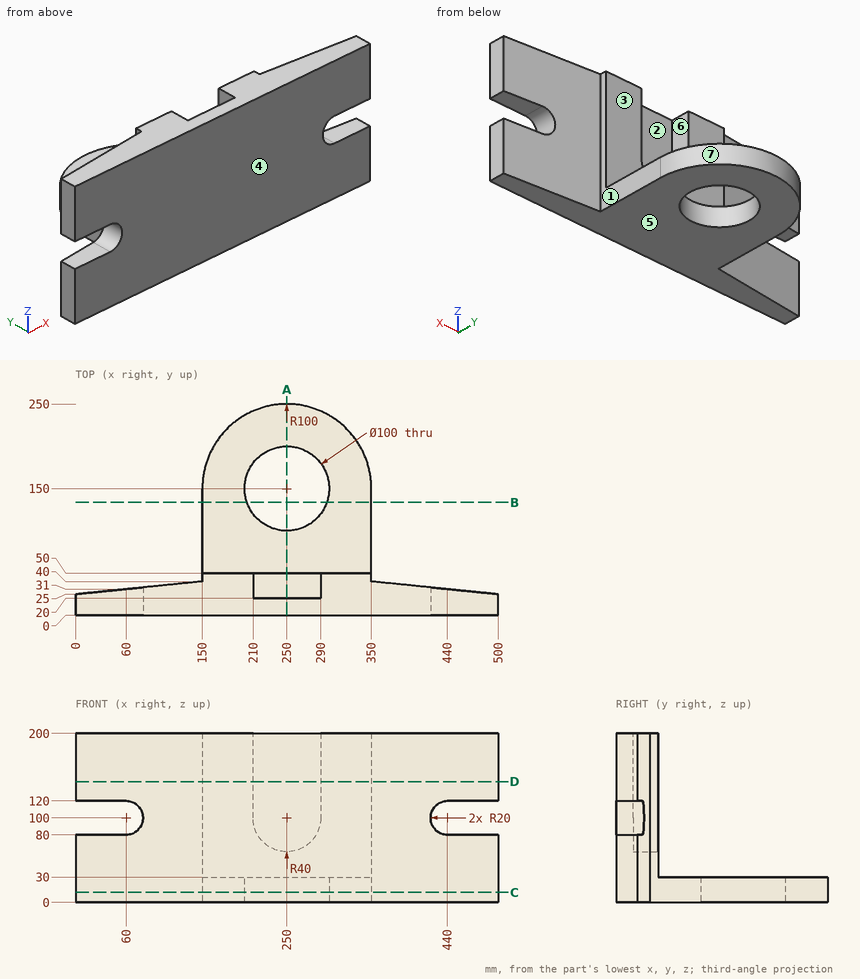
Here's the drawing with two shaded views (mm, measured from the low corner). I have some questions. A direction names the side the tool comes from. Give positions to 0.01 mm unless a question says otherwise; leave off trailing zeros. Write each loop counter-clockwise with the first axis right and the second up, starting at its lowest first coordinate (ties: lowest second). Pieces come first, ordered by that corner, then holes. Notation, with made-up numbers: (-23, 33) - (1, 33) arc R27 ccw to (1, 49) - close; hole circle Ø1 at (42, 55). An arc over 180 degrees is marked (long way). One line per item, written item: value. Start each with the question number.
Item 1: I'm going to push flat-ended pins straight in: pin 1 (8 mm diameter, centred on y = 68.5, z = 29.5, fed in from +X); pin 2 (3 mm diameter, centred on x = 187.5, z = 29.5, fed in from +Y). Where does each tip first touch, or does it pass through?
Item 2: Which directions (+Z, -Z, +X, -X, +Y, -Y) give clear straight access to the entire face, cutting with the end or side of a thin tool? Please do the marked faces 1, 2, 3 and 4.
Item 3: Imagine slicing it at B-B, the plane y = 133.5. List the corners of the cut face in (x, z) for me, and give its area (3 significant figures).
Item 4: Imagine slicing it at D-D, the plane z = 143. List the corners of the cut face in (x, y) for me, and give its area (4 significant figures).
Item 5: Imagine slicing it at C-C, the plane z = 12. List the corners of the cut face in (x, y) for me.
Item 6: Imagine slicing it at A-A, the plane x = 250. List the corners of the cut face in (y, z) for me.
Item 7: If we mould it in two halves opening along X, with no side actions, what happens to the marked faces 5, 6 and 7? For each: +X half, -X half, draft (parallel to the pull), parting line (faces both ways), or undercut.
Item 8: Please list where these lines run through material, in increasing order: line 1 (Y direction, x = 250, z = 8); line 2 (Z direction, x = 220, y = 83); line 3 (Z direction, x = 38, y = 16). Write a range as from..to.
Geometry says:
1. pin 1: x = 350
1. pin 2: y = 229.24
2. face 1: +Z, -Z, +X, +Y
2. face 2: +Z, +Y
2. face 3: +Z, +X, -X, +Y
2. face 4: +Z, -Z, +X, -X, -Y
3. outline: (150, 0) - (202.8, 0) - (202.8, 30) - (150, 30) - close; (297.2, 0) - (350, 0) - (350, 30) - (297.2, 30) - close
3. area: 3,170 mm^2
4. outline: (0, 0) - (500, 0) - (500, 25) - (350, 40) - (350, 50) - (290, 50) - (290, 20) - (210, 20) - (210, 50) - (150, 50) - (150, 40) - (0, 25) - close
4. area: 17,350 mm^2
5. outline: (0, 0) - (500, 0) - (500, 25) - (350, 40) - (350, 150) arc R100 ccw to (150, 150) - (150, 40) - (0, 25) - close; hole circle Ø100 at (250, 150)
6. outline: (0, 0) - (100, 0) - (100, 30) - (50, 30) - (50, 60) - (20, 60) - (20, 200) - (0, 200) - close; (200, 0) - (250, 0) - (250, 30) - (200, 30) - close
7. face 5: draft
7. face 6: undercut
7. face 7: parting line
8. line 1: 0..100, 200..250
8. line 2: 0..30
8. line 3: 0..80, 120..200
